```python
from build123d import *

# Parameters (mm, degrees)
F0_W     = 45
F0_H     = 50
F1_DEPTH = 110
F2_W     = 45
F2_H     = 50
F3_DEPTH = 70
F4_R     = 5
F5_W     = 5
F5_H     = 30
F6_DEPTH = 17
F7_R     = 7.5
F7_R_2   = 5
F8_DEPTH = 25


with BuildPart() as f1:
    # F0 (on Top) → F1 (new body)
    with BuildSketch(Plane.XY):
        Rectangle(F0_W, F0_H)
    extrude(amount=F1_DEPTH)

    # F2 (on face) → F3 (join)
    with BuildSketch(Plane.XY.offset(110)):
        with BuildLine():
            ThreePointArc((-27.5, -25), (-26.0355339059, -28.5355339059), (-22.5, -30))
            Line((-22.5, -30), (22.5, -30))
            ThreePointArc((22.5, -30), (26.0355339059, -28.5355339059), (27.5, -25))
            Line((27.5, -25), (27.5, 25))
            ThreePointArc((27.5, 25), (26.0355339059, 28.5355339059), (22.5, 30))
            Line((22.5, 30), (-22.5, 30))
            ThreePointArc((-22.5, 30), (-26.0355339059, 28.5355339059), (-27.5, 25))
            Line((-27.5, 25), (-27.5, -25))
        make_face()
        Rectangle(F2_W, F2_H, mode=Mode.SUBTRACT)
        Rectangle(F2_W, F2_H)
    extrude(amount=F3_DEPTH)

    # F4
    f4_edges = [f1.edges().sort_by_distance(p)[0] for p in [
        (22.5, 25, 55),
        (22.5, -25, 55),
        (-22.5, -25, 55),
        (-22.5, 25, 55),
    ]]
    fillet(f4_edges, radius=F4_R)

    # F5 (on face) → F6 (cut)
    with BuildSketch(Plane.XZ.offset(25)):
        with Locations((-12, 19)):
            Rectangle(F5_W, F5_H)
        with Locations((-4, 19)):
            Rectangle(F5_W, F5_H)
        with Locations((4, 19)):
            Rectangle(F5_W, F5_H)
        with Locations((12, 19)):
            Rectangle(F5_W, F5_H)
    extrude(amount=-F6_DEPTH, mode=Mode.SUBTRACT)

    # F7 (on face) → F8 (join)
    with BuildSketch(Plane.XZ.offset(30)):
        with Locations((0, 160)):
            Circle(F7_R)
        with Locations((0, 160)):
            Circle(F7_R_2, mode=Mode.SUBTRACT)
    extrude(amount=F8_DEPTH)


solid = f1.part
```
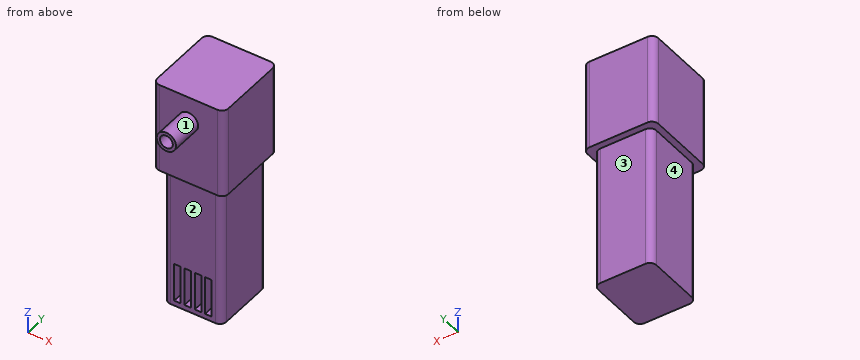
Source: CAD feature listing. Evaluate the final solid. Frame: model axes, mm. Face numbers are marked on the shaded views. A direction names the side the tool comes from. Round coordinates to 2 decimals unless told otherwise and drop trailing zeros. Loops run counter-clockwise (first coordinate to the right, second up) from the corner with the lowest first, then second, coordinate; pieces in that order, holes last. Notation, with made-up numbers: M 37,4 L 45,4 A19 cw 45,26 Z; hole C -11,86.25 d10. An arc over 180 degrees is marked long. Use a Markdown table: item, result. Add a question column.
1. Section query C-C on z = 62. Return the cut outline in (x, y).
2. Reachability of the marked faces 1, 2, 3 and 4 from +Z, -Z, +X, -X, +Y, -Y: full face, straight path, thin tool, end or side. Return the list, or none.
3. Line query: line 1 (Z direction, x = 0, y = -42.5); line 2 (Y direction, x = 12.5, z = 137.5); line 3 (X direction, y = -6, z = 84). Output: solid intervals per line, ascending.
4. Section query B-B on z = 150. Return the cut outline in (x, y), then the cut area to 3 significant figures.
5. Section query A-A on y = -11.5. Return the cut outline in (x, z), then the cut area to 3 significant figures.
6. Section query D-D on y = -37. Return the cut outline in (x, z), then the cut area to 3 significant figures.
7. Contact query for flat-ended pins moving along their axis: P1, Ø18.5, axis at y = -12.5, z = 23.5, coming from the +X side; P2, Ø18.5, axis at y = -16.5, z = 21, coming from the -X side; P3, Ø10, axis at x = 5.5, y = -30.5, coming from the +Z side; P4, Ø8, axis at x = -2, z = 77, coming from the -Y side. Output: stop coordinate, or through.
Reported:
| question | item | result |
|---|---|---|
| 1 | outline | M -22.5,-20 A5 ccw -17.5,-25 L 17.5,-25 A5 ccw 22.5,-20 L 22.5,20 A5 ccw 17.5,25 L -17.5,25 A5 ccw -22.5,20 Z |
| 2 | face 1 | -Y |
| 2 | face 2 | -Z, +X, -X, -Y |
| 2 | face 3 | -Z, +X, -X, +Y |
| 2 | face 4 | -Z, -X, +Y, -Y |
| 3 | line 1 | z = 152.5 to 155, 165 to 167.5 |
| 3 | line 2 | y = -30 to 30 |
| 3 | line 3 | x = -22.5 to 22.5 |
| 4 | outline | M -27.5,-25 A5 ccw -22.5,-30 L 22.5,-30 A5 ccw 27.5,-25 L 27.5,25 A5 ccw 22.5,30 L -22.5,30 A5 ccw -27.5,25 Z |
| 4 | area | 3,280 mm² |
| 5 | outline | M -27.5,110 L -22.5,110 L -22.5,0 L 22.5,0 L 22.5,110 L 27.5,110 L 27.5,180 L -27.5,180 Z; hole M -14.5,4 L -9.5,4 L -9.5,34 L -14.5,34 Z; hole M -6.5,4 L -1.5,4 L -1.5,34 L -6.5,34 Z; hole M 1.5,4 L 6.5,4 L 6.5,34 L 1.5,34 Z; hole M 9.5,4 L 14.5,4 L 14.5,34 L 9.5,34 Z |
| 5 | area | 8,200 mm² |
| 6 | outline | C 0,160 d15; hole C 0,160 d10 |
| 6 | area | 98.2 mm² |
| 7 | P1 | stops at x = 22.5 |
| 7 | P2 | stops at x = -22.5 |
| 7 | P3 | stops at z = 180 |
| 7 | P4 | stops at y = -25 |
